Work out the finished part from the listing and answer in its coordinate system (mm). A direction names the side the tool comes from. Round coordinates to 2 decimals unless told otherwise and drop trailing zeros. Loops run counter-clockwise (first coordinate to the right, second up) from the corner with the lowest first, then second, coordinate; pieces in that order, holes last. Notation, with made-up numbers: (-26, 42) -> (-18, 42) arc R11 ccw to (-18, 61) -> close; hole circle Ø11 at (33, 16). An arc over 180 degrees is marked (long way). Use one line per item in the form item = value.
```python
from build123d import *

# Parameters (mm, degrees)
BOSS_EXTRUDE1_DEPTH     = 3.175
CUT_EXTRUDE1_DEPTH      = 16.968703454
CUT_EXTRUDE1_DEPTH_BACK = 16.968703454
SKETCH4_W               = 2.032
SKETCH4_H               = 12.7


with BuildPart() as part:
    # Sketch1 → Boss-Extrude1 (new, symmetric)
    with BuildSketch(Plane.XY):
        Polygon((0, 0), (9.652, 0), (9.652, 2.794), (7.62, 2.794), (7.62, 5.969), (2.032, 5.969), (2.032, 2.794), (0, 2.794), align=None)
    extrude(amount=BOSS_EXTRUDE1_DEPTH, both=True)

    # Sketch3 → Revolve1 (revolve)
    with BuildSketch(Plane.XY, mode=Mode.PRIVATE) as revolve1_sk:
        Polygon((3.76219647, 12.319), (4.326476153, 12.319), (4.326476153, 5.969), (2.286, 5.969), (2.286, 10.6045), (1.778, 11.38048125), align=None)
    revolve(revolve1_sk.sketch.rotate(Axis((4.826, 5.969, 0), (0, 1, 0)), 270), axis=Axis((4.826, 5.969, 0), (0, 1, 0)))

    # Sketch4 → Cut-Extrude1 (cut, two sides: drawn at the far end of the back side and taken through both)
    with BuildSketch(Plane.XY.offset(-CUT_EXTRUDE1_DEPTH_BACK)):
        with Locations((4.826, 12.319)):
            Rectangle(SKETCH4_W, SKETCH4_H)
    extrude(amount=CUT_EXTRUDE1_DEPTH + CUT_EXTRUDE1_DEPTH_BACK, mode=Mode.SUBTRACT)


solid = part.part
```
(1) Find section A-A, the plane z = 0. Write down the section's boundary in (x, y).
Completed:
outline = (0, 0) -> (9.65, 0) -> (9.65, 2.79) -> (7.62, 2.79) -> (7.62, 5.97) -> (7.37, 5.97) -> (7.37, 10.6) -> (7.87, 11.38) -> (5.89, 12.32) -> (5.84, 12.32) -> (5.84, 5.97) -> (3.81, 5.97) -> (3.81, 12.32) -> (3.76, 12.32) -> (1.78, 11.38) -> (2.29, 10.6) -> (2.29, 5.97) -> (2.03, 5.97) -> (2.03, 2.79) -> (0, 2.79) -> close
(2) Consider L1, parallel to X at y = 4.5, z = 0; L2, parallel to Y at x = 4.25, z = 2.75; L3, parallel to Y at x = 1, z = -1.25. Determine where each line is inside the solid, lowest interval first.
Completed:
L1 = 2.03 to 7.62
L2 = 0 to 5.97
L3 = 0 to 2.79
(3) Find section B-B, the plane y = 10. Write down the section's boundary in (x, z).
Completed:
outline = (3.81, -2.33) -> (3.81, 2.33) arc R2.54 ccw to start; (5.84, -2.33) arc R2.54 ccw to (5.84, 2.33) -> close
(4) Given P1, Ø2, axis at y = 10.5, z = 0, coming from the -X side; P2, Ø1, axis at x = 5.5, z = -2, coming from the +Y side; P3, Ø1.6, axis at y = 5, z = 1.5, coming from the +X side, each flat-ended and moving along its own axis, determine where each tip first touches the part or whether it passes through.
Completed:
P1 = 1.78
P2 = 11.91
P3 = 7.62
(5) For faces 1 (the flat face through (7.62, 4, 0)), 2 (the cylindrical face through (2.286, 8.319, -0.041)), 3 (the conical face through (7.454, 10.739, 0.045)), 4 (the flat face through (2.032, 4, 0)), 5 (the flat face through (3.81, 9, 0)), determine the directions among +Z, -Z, +X, -X, +Y, -Y from which every point of the face is accessible in a straight line to the end or side of a thin tool.
Completed:
face_1 = +Z, -Z, +X
face_2 = -X
face_3 = +X
face_4 = +Z, -Z, -X
face_5 = +Z, -Z, +Y
(6) Find section D-D, the plane y = 5.25. Write down the section's boundary in (x, z) (3 decimals), then the cut area to 3 significant figures.
Completed:
outline = (2.032, -3.175) -> (7.62, -3.175) -> (7.62, 3.175) -> (2.032, 3.175) -> close
area = 35.5 mm2
(7) For a pull along X with two mould halves and no side action, classify faces 6 (the flat face through (5.842, 9, 0)), 7 (the cylindrical face through (7.366, 8.319, 0.041)), 8 (the conical face through (3, 11.96, -0.03)) as +X half, -X half, draft (parallel to the pull), parting line (faces both ways), or undercut.
Completed:
face_6 = undercut
face_7 = +X half
face_8 = -X half
(8) Find section C-C, the plane x = 5.25. Write down the section's boundary in (y, z) (3 decimals).
Completed:
outline = (0, -3.175) -> (5.969, -3.175) -> (5.969, 3.175) -> (0, 3.175) -> close
